Here's how the part is built. I have some questions about the finished solid (model axes, mm). A direction names the side the tool comes from. Give positions to 0.01 mm unless a question says otherwise; leave off trailing zeros. Loops run counter-clockwise (first coordinate to the right, second up) from the corner with the lowest first, then second, coordinate; pieces in that order, holes last. Notation, with made-up numbers: (48, -2) - (71, -2) arc R24 ccw to (71, 8) - close; hole circle Ø4 at (-21.5, 28). An arc over 180 degrees is marked (long way). Use one line per item in the form item = value.
from build123d import *

# Parameters (mm, degrees)
SKETCH1_W                = 41
SKETCH1_H                = 45
BOSS_EXTRUDE1_DEPTH      = 2
SKETCH3_W                = 41
SKETCH3_H                = 2
BOSS_EXTRUDE2_DEPTH      = 10
SKETCH9_W                = 2
SKETCH9_H                = 48.933806043
BOSS_EXTRUDE6_DEPTH      = 10
SKETCH7_W                = 41
SKETCH7_H                = 1.933806043
BOSS_EXTRUDE7_DEPTH      = 8
BOSS_EXTRUDE7_DEPTH_BACK = 2
SKETCH10_W               = 2.62804999
SKETCH10_H               = 48.933806043
BOSS_EXTRUDE8_DEPTH      = 10
FILLET3_R                = 5
FILLET4_R                = 2


with BuildPart() as part:
    # Sketch1 → Boss-Extrude1 (new body)
    with BuildSketch(Plane(origin=(0, 0, 0), x_dir=(1, 0, 0), z_dir=(0, 1, 0))):
        with Locations((0.11627907, -1.098837209)):
            Rectangle(SKETCH1_W, SKETCH1_H)
    extrude(amount=BOSS_EXTRUDE1_DEPTH)

    # Sketch3 → Boss-Extrude2 (add)
    with BuildSketch(Plane(origin=(0, 2, 0), x_dir=(1, 0, 0), z_dir=(0, 1, 0))):
        with Locations((0.11627907, -24.598837209)):
            Rectangle(SKETCH3_W, SKETCH3_H)
    extrude(amount=-BOSS_EXTRUDE2_DEPTH)

    # Sketch9 → Boss-Extrude6 (add)
    with BuildSketch(Plane(origin=(0, 2, 0), x_dir=(1, 0, 0), z_dir=(0, 1, 0))):
        with Locations((-21.38372093, -1.131934188)):
            Rectangle(SKETCH9_W, SKETCH9_H)
    extrude(amount=-BOSS_EXTRUDE6_DEPTH)

    # Sketch7 → Boss-Extrude7 (add, two sides)
    with BuildSketch(Plane(origin=(0, 0, 0), x_dir=(-1, 0, 0), z_dir=(0, -1, 0))) as boss_extrude7_sk:
        with Locations((-0.11627907, 22.368065812)):
            Rectangle(SKETCH7_W, SKETCH7_H)
    extrude(amount=BOSS_EXTRUDE7_DEPTH)
    extrude(boss_extrude7_sk.sketch, amount=-BOSS_EXTRUDE7_DEPTH_BACK)

    # Sketch10 → Boss-Extrude8 (add)
    with BuildSketch(Plane(origin=(0, -8, 0), x_dir=(-1, 0, 0), z_dir=(0, -1, 0))):
        with Locations((-21.930304065, -1.131934188)):
            Rectangle(SKETCH10_W, SKETCH10_H)
    extrude(amount=-BOSS_EXTRUDE8_DEPTH)

    # Fillet3
    fillet3_edges = [part.edges().sort_by_distance(p)[0] for p in [
        (0.430304065, 2, 25.598837209),
        (-22.38372093, -3, 25.598837209),
        (-22.38372093, -3, -23.334968834),
        (0.430304065, 2, -23.334968834),
        (-22.38372093, 2, 1.131934188),
        (23.24432906, 2, 1.131934188),
        (23.24432906, -3, 25.598837209),
        (23.24432906, -3, -23.334968834),
    ]]
    fillet(fillet3_edges, radius=FILLET3_R)

    # Fillet4
    fillet4_edges = [part.edges().sort_by_distance(p)[0] for p in [
        (-20.38372093, -4, 23.598837209),
        (20.61627907, -4, 23.598837209),
        (-20.38372093, -4, -21.401162791),
        (20.61627907, -4, -21.401162791),
    ]]
    fillet(fillet4_edges, radius=FILLET4_R)


solid = part.part
(1) For P1, Ø3, axis at y = -2.5, z = -7.5, coming from the +X side; P2, Ø4, axis at x = -14.5, z = -3, coming from the -Y side; P3, Ø3, axis at y = -1, z = -13.5, coming from the -X side; P4, Ø2, axis at y = 0.5, z = -11, coming from the +X side, each with a flat end and sliding along its axis, tell me the tip position at first contact or that it passes through.
Geometry says:
P1 = 23.24
P2 = 0
P3 = -22.36
P4 = 22.57
(2) Thinking about a two-plate mould opening in X: for faces 1 (the flat face through (0, -4, 23.599)), 2 (the cylindrical face through (-19.81, -4.06, 23)), 3 (the cylindrical face through (21.819, 0.496, 0.859)), 4 (the cylindrical face through (-20.88, 0.574, 0.859)), which applies, pulls with the +X half, pulls with the -X half, needs draft (parallel to the pull), parting line crosses it, or undercut?
Geometry says:
face_1 = undercut
face_2 = undercut
face_3 = pulls with the +X half
face_4 = pulls with the -X half
(3) If we section it at C-C (y = -6.5): List the corners of the cut face in (x, z) for me.
Geometry says:
outline = (-22.38, -18.33) arc R5 ccw to (-17.38, -23.33) - (18.24, -23.33) arc R5 ccw to (23.24, -18.33) - (23.24, 20.6) arc R5 ccw to (18.24, 25.6) - (-17.38, 25.6) arc R5 ccw to (-22.38, 20.6) - close; hole (-20.38, -19.4) arc R2 ccw to (-18.38, -21.4) - (18.62, -21.4) arc R2 ccw to (20.62, -19.4) - (20.62, 21.6) arc R2 ccw to (18.62, 23.6) - (-18.38, 23.6) arc R2 ccw to (-20.38, 21.6) - close
(4) If we section it at B-B (x = 6): List the corners of the cut face in (y, z) for me, plus the area to 3 significant figures.
Geometry says:
outline = (-8, -23.33) - (-3, -23.33) arc R5 ccw to (2, -18.33) - (2, 20.6) arc R5 ccw to (-3, 25.6) - (-8, 25.6) - (-8, 23.6) - (0, 23.6) - (0, -21.4) - (-8, -21.4) - close
area = 119 mm²
(5) If we section it at A-A (z = 14): List the corners of the cut face in (x, y) for me, plus the area to 3 significant figures.
Geometry says:
outline = (-22.38, -8) - (-20.38, -8) - (-20.38, 0) - (20.62, 0) - (20.62, -8) - (23.24, -8) - (23.24, -3) arc R5 ccw to (18.24, 2) - (-17.38, 2) arc R5 ccw to (-22.38, -3) - close
area = 118 mm²
(6) If we section it at D-D (y = 1): List the corners of the cut face in (x, z) for me.
Geometry says:
outline = (-20.38, -18.33) arc R3 ccw to (-17.38, -21.33) - (18.24, -21.33) arc R3 ccw to (21.24, -18.33) - (21.24, 20.6) arc R3 ccw to (18.24, 23.6) - (-17.38, 23.6) arc R3 ccw to (-20.38, 20.6) - close
(7) For faces 5 (the cylindrical face through (21.819, -5.465, 24.095)), 6 (the flat face through (0, -4, -21.401)), which set-ups out of +Z, -Z, +X, -X, +Y, -Y let a thin tool reach every point of the face, with its end or its side?
Geometry says:
face_5 = +Z, +X, +Y, -Y
face_6 = -Y
(8) If I drill on probe 1 along Z at (x, y) = (-17.5, -4.75); probe 2 along X at (y, z) = (-3.5, -17); probe 3 along Y at (x, z) = (-16, 17.5), over which ranges is the centre line in solid material (lowest first)?
Geometry says:
probe_1 = -23.33 to -21.4, 23.6 to 25.6
probe_2 = -22.38 to -20.38, 20.62 to 23.24
probe_3 = 0 to 2
